Autodesk Inventor part; units mm, degrees
ref_plane "YZ Plane" through (0, 0, 0) normal (1, 0, 0) x (0, 1, 0)
ref_plane "XZ Plane" through (0, 0, 0) normal (0, 1, 0) x (-1, 0, 0)
ref_plane "XY Plane" through (0, 0, 0) normal (0, 0, 1) x (1, 0, 0)
sketch "Sketch1" plane through (0, 0, 0) normal (0, 0, 1) x (1, 0, 0)
  circle A0 centre (0, 0) radius 12
  circle A1 centre (0, 0) radius 15.175
  dimension "d0" = 24
  dimension "d1" = 3.175
extrude "Extrusion1" add sketch "Sketch1" along normal mid plane 100
sketch "Sketch2" plane through (0, 0, 0) normal (0, 1, 0) x (-1, 0, 0)
  line L0 (15.175, -50) -> (15.175, 50)
  line L1 (-12, -50) -> (-12, 50)
  line L2 (-15.175, -50) -> (-15.175, 50)
  line L3 (15.175, 12.7) -> (15.175, -12.7)
  line L4 (0, -70) -> (0, 70)
  line L5 (-12, -50) -> (-12, 50)
  line L6 (-12, -9.525) -> (-15.175, -9.525)
  line L7 (-15.175, -9.525) -> (-15.175, 9.525)
  line L8 (-15.175, 9.525) -> (-12, 9.525)
  line L9 (-12, 9.525) -> (-12, -9.525)
  point P0 (0, 0)
  point P1 (12, 0)
  point P2 (-12, 0)
  dimension "d6" = 19.05
revolve "Revolution1" cut sketch "Sketch2" angle 120 mid plane about axis through (0, 0, -10) along (0, 0, 1)
sketch "Sketch4" plane through (0, 0, 0) normal (0, 0, 1) x (1, 0, 0)
  arc A0 (6.8593, 9.8463) -> (6.8593, -9.8463) centre (0, 0) ccw
  arc A1 (6.8593, 9.8636) -> (6.8593, -9.8636) centre (0, 0) ccw
  line L0 (6.8593, 9.8636) -> (6.8593, 9.8463)
  line L1 (6.8593, -9.8463) -> (6.8593, -9.8636)
  dimension "d9" = 24.0284
extrude "Extrusion2" cut sketch "Sketch4" along normal mid plane 76.2
properties part number "DPLX_P033_SG_Viton rubber Cover" material "Rubber, Silicone"
The model under review builds one solid part; all positions refer to its coordinate system, in mm. A direction names the side the tool comes from. Round coordinates to 2 decimals unless told otherwise and drop trailing zeros. Write each loop counter-clockwise with the first axis right and the second up, starting at its lowest first coordinate (ties: lowest second). Pieces come first, ordered by that corner, then holes. Notation, with made-up numbers: (73.5, -30.75) -> (97.5, -30.75) arc R15 ccw to (97.5, -8.75) -> close; hole circle Ø2 at (31, 76.5). An arc over 180 degrees is marked (long way). Use CSV: the item, a comma, the result in double quotes.
Q1. For pin 1 Ø3 at (x, z) = (4.5, 1.5) entering from +Y; pin 2 Ø4 at (y, z) = (-4, -38) entering from +X; pin 3 Ø1 at (x, z) = (4, -22.5) entering from +Y, all flat-tipped, find the tip position at first contact; note any pin that passes through.
Checks:
pin 1,"y = 14.88"
pin 2,"x = 15.04"
pin 3,"y = 14.77"
Q2. Mouldability with a two-part tool opening along Z and no side actions: class faces 1 (the flat face through (12.2, -0.2, -9.525)), 2 (the flat face through (10, -7, -50)) as released by +Z, released by -Z, zero draft, split by the parting line, or undercut.
Checks:
face 1,"undercut"
face 2,"released by -Z"
Q3. Consider section B-B (y = 0). Give the boundary of the cut face in (x, z) (3 decimals), then the cut area to 3 significant figures.
Checks:
outline,"(-15.175, -50) -> (-12, -50) -> (-12, -38.1) -> (-12.014, -38.1) -> (-12.014, 38.1) -> (-12, 38.1) -> (-12, 50) -> (-15.175, 50) -> close; (12, -50) -> (15.175, -50) -> (15.175, -9.525) -> (12, -9.525) -> close; (12, 9.525) -> (15.175, 9.525) -> (15.175, 50) -> (12, 50) -> close"
area,"573 mm²"
Q4. Consider section C-C (z = 23). Give the boundary of the cut face in (x, y) (3 decimals), then the cut area to 3 significant figures.
Checks:
outline,"circle Ø30.35 at (0, 0); hole (6.859, -9.864) -> (6.859, -9.846) arc R12 ccw to (6.859, 9.846) -> (6.859, 9.864) arc R12.014 ccw (long way) to start"
area,"270 mm²"
Q5. To check wall thickness, follow probe 1 along Z at (x, y) = (13.5, 6.5) (3 decimals); probe 2 along Y at (x, z) = (0, 38.5) (3 decimals); probe 3 along Y at (x, z) = (-4, 36). State the ranges of each line that lie inside material, in increasing order. Write a range as [from, to].
Checks:
probe 1,"[-50, -9.525], [9.525, 50]"
probe 2,"[-15.175, -12], [12, 15.175]"
probe 3,"[-14.64, -11.33], [11.33, 14.64]"
Q6. For faces 3 (the cylindrical face through (11.446, 3.604, -38.474)), 4 (the flat face through (6.808, -11.792, 0.133)), list the 3-axis set-ups (+Z, -Z, +X, -X, +Y, -Y) from which the entire face can be reached by the end or side of a thin tool; tool diameter is ignored.
Checks:
face 3,"+Z, -Z"
face 4,"+X"
